```python
from build123d import *

# Parameters (mm, degrees)
SKETCH1_W           = 60.96
SKETCH1_H           = 60.96
SKETCH1_R           = 2.4765
BOSS_EXTRUDE3_DEPTH = 76.2
SKETCH3_R           = 3.175
BOSS_EXTRUDE4_DEPTH = 50.8


with BuildPart() as part:
    # Sketch1 → Boss-Extrude3 (new body)
    with BuildSketch(Plane(origin=(0, 0, 0), x_dir=(0, 0, -1), z_dir=(1, 0, 0))):
        Rectangle(SKETCH1_W, SKETCH1_H)
        with Locations((-23.573172318, 23.573172318)):
            Circle(SKETCH1_R, mode=Mode.SUBTRACT)
        with Locations((23.573172318, 23.573172318)):
            Circle(SKETCH1_R, mode=Mode.SUBTRACT)
        with Locations((23.573172318, -23.573172318)):
            Circle(SKETCH1_R, mode=Mode.SUBTRACT)
        with Locations((-23.573172318, -23.573172318)):
            Circle(SKETCH1_R, mode=Mode.SUBTRACT)
    extrude(amount=BOSS_EXTRUDE3_DEPTH)

    # Sketch3 → Boss-Extrude4 (add)
    with BuildSketch(Plane.ZY):
        Circle(SKETCH3_R)
    extrude(amount=BOSS_EXTRUDE4_DEPTH)


solid = part.part
```
Verification items for the finished model (mm, model axes). A direction names the side the tool comes from. Give positions to 0.01 mm unless a question says otherwise; leave off trailing zeros. Order: outer loops, then holes, each group sorted by start corner. A loop starts at its lowest first (then second) coordinate and runs counter-clockwise, first axis right, second up. Notation, with made-up numbers: M -7,58.5 L 23,58.5 A3 cw 23,62.5 Z; hole C 34.5,31.5 d3. An arc over 180 degrees is marked long. Answer in a Markdown table with one row per item. Add a question column.
Item 1: Mould release check, pull along Y, two halves, no side actions. Record for faces 3 (the flat face through (38, 30.48, 0)), 4 (the flat face through (76.2, 0, 0)), 5 (the cylindrical face through (37.567, 25.661, -24.905)): released by +Y, released by -Y, zero draft, split by the parting line, or undercut.
Item 2: Tool access check on faces 1 (the cylindrical face through (37.57, 26.03, 23.9)), 2 (the cylindrical face through (-25.04, -3.1, -0.69)). Record the directions out of +Z, -Z, +X, -X, +Y, -Y that give a thin tool (end or side, any length) a straight path to the whole face; none if there is none.
Item 3: Scan lines: probe 1 along Z at (x, y) = (27.5, -23.5); probe 2 along Z at (x, y) = (14, -22.5); probe 3 along X at (y, z) = (-9, 11.5). Record each from-to range of solid material in increasing order. Write a range as from..to.
Item 4: Section check B-B, the plane y = 0. Enter the section's corners in (x, z) (3 decimals).
Item 5: Gauge pin test, flat end, axial feed: pin 1 (8 mm diameter, centred on y = -13.5, z = 22, fed in from -X). Record the tip position at first contact, or that the pin passes through.
Item 6: Section check A-A, the plane z = -23. Enter the section's corners in (x, y), and give its area (3 significant figures).
Item 7: Section check C-C, the plane x = 31. Enter the section's corners in (y, z), and give its area (3 significant figures).
Filled sheet:
| question | item | result |
|---|---|---|
| 1 | face 3 | released by +Y |
| 1 | face 4 | zero draft |
| 1 | face 5 | undercut |
| 2 | face 1 | +X, -X |
| 2 | face 2 | -X |
| 3 | probe 1 | z = -30.48..-26.05, -21.1..21.1, 26.05..30.48 |
| 3 | probe 2 | z = -30.48..-25.81, -21.34..21.34, 25.81..30.48 |
| 3 | probe 3 | x = 0..76.2 |
| 4 | outline | M -50.8,-3.175 L 0,-3.175 L 0,-30.48 L 76.2,-30.48 L 76.2,30.48 L 0,30.48 L 0,3.175 L -50.8,3.175 Z |
| 5 | pin 1 | stops at x = 0 |
| 6 | outline | M 0,-30.48 L 76.2,-30.48 L 76.2,-25.98 L 0,-25.98 Z; M 0,-21.16 L 76.2,-21.16 L 76.2,21.16 L 0,21.16 Z; M 0,25.98 L 76.2,25.98 L 76.2,30.48 L 0,30.48 Z |
| 6 | area | 3,910 mm^2 |
| 7 | outline | M -30.48,-30.48 L 30.48,-30.48 L 30.48,30.48 L -30.48,30.48 Z; hole C -23.57,-23.57 d4.95; hole C -23.57,23.57 d4.95; hole C 23.57,-23.57 d4.95; hole C 23.57,23.57 d4.95 |
| 7 | area | 3,640 mm^2 |
